Here's how the part is built. I have some questions about the finished solid (model axes, mm). A direction names the side the tool comes from. Give positions to 0.01 mm unless a question says otherwise; leave off trailing zeros. Loops run counter-clockwise (first coordinate to the right, second up) from the corner with the lowest first, then second, coordinate; pieces in that order, holes last.
Q1. I need wall thicknesses on probe 1 along X at (y, z) = (-45, -8); probe 2 along Y at (x, z) = (41, -0.5); probe 3 along Z at (x, y) = (-34, 45). Which ranges of each line are inside material? Lowest first, please.
Q2. Suppose I cut it at A-A (y = -44). List the corners of the cut face in (x, z) for me, and give its area (3 significant figures).
Q3. I'm going to push flat-ended pins straight in: P1, Ø7, axis at y = 15.5, z = -0.5, coming from the +X side; P2, Ø10, axis at x = -50, y = 1.5, coming from the +Z side; P3, Ø6.5, axis at y = -75.5, z = 1, coming from the -X side. Where does each tip first touch, or does it pass through?
Q4. Thinking about a two-plate mould opening in Y: for faces 1 (the face through (69.85, -76, 0)), 2 (the face through (57.15, 15, 0)), 3 (the face through (67.63, -74.75, -12.28)), 4 (the face through (1.2, 61.1, -5.6)), which applies, pulls with the +Y half, pulls with the -Y half, needs draft (parallel to the pull), parting line crosses it, or undercut?
Q5. For faces 5 (the face through (34.436, -78.468, -1.816)), 6 (the face through (58.402, 12.9, 2.146)), 7 (the face through (0.212, -74.751, -23.872)), 8 (the face through (-69.02, -36.06, -23.95)), 9 (the face through (-1, -63.5, -6)), which set-ups out of +Z, -Z, +X, -X, +Y, -Y let a thin tool reach every point of the face, with its end or its side?
```python
from build123d import *

# Parameters (mm, degrees)
F4_DEPTH       = 25.4
F1_R           = 6.35
F5_DEPTH       = 69.85
F3_R           = 6.604
F6_DEPTH       = 69.85
F7_R           = 5.07999
F2_R           = 2.9845
F8_DEPTH       = 69.85
F10_DEPTH      = 11.43
F12_DEPTH      = 25.4
F12_DEPTH_BACK = 25.4
F13_R          = 3.175
F14_DEPTH      = 59.69
F14_DEPTH_BACK = 59.69
F15_R          = 3.1877
F16_DEPTH      = 57.15
F16_DEPTH_BACK = 57.15


# Not quite as in the source:
# - a fillet or chamfer is up to 0.001 mm smaller than in the source, because OpenCascade refuses the exact size


with BuildPart() as f4:
    # F0 (on Top) → F4 (new body)
    with BuildSketch(Plane.XY):
        with BuildLine():
            Line((69.1548068551, -76.2), (69.1548068551, 0))
            ThreePointArc((69.1548068551, 0), (-0.6951931449, 69.85), (-70.5451931449, 0))
            Line((-70.5451931449, 0), (-70.5451931449, -76.2))
            Line((-70.5451931449, -76.2), (69.1548068551, -76.2))
        make_face()
    extrude(amount=-F4_DEPTH)

    # F1 (on Right) → F5 (join)
    with BuildSketch(Plane.YZ):
        with Locations((-76.4005258679, 0)):
            Circle(F1_R)
    extrude(amount=-F5_DEPTH)

    # F3 (on Right) → F6 (cut)
    with BuildSketch(Plane.YZ):
        with Locations((-76.365634799, 0)):
            Circle(F3_R)
    extrude(amount=F6_DEPTH, mode=Mode.SUBTRACT)

    # F7 (radius 5.08 in the source; OpenCascade refuses exactly that, so slightly less here)
    f7_edges = [f4.edges().sort_by_distance(p)[0] for p in [
        (-0.695193, -76.2, -25.4),
        (-70.545193, -38.1, -25.4),
        (-70.545193, -76.2, -12.7),
        (69.154807, -76.2, -16.000961),
    ]]
    fillet(f7_edges, radius=F7_R)

    # F2 (on Right) → F8 (join)
    with BuildSketch(Plane.YZ):
        with Locations((-76.0997384787, 0)):
            Circle(F2_R)
    extrude(amount=F8_DEPTH)

    # F9 (on Top) → F10 (cut)
    with BuildSketch(Plane.XY):
        with BuildLine():
            Line((60.994354069, -63.5), (60.994354069, 0))
            ThreePointArc((60.994354069, 0), (-0.118045931, 61.1124), (-61.230445931, 0))
            Line((-61.230445931, 0), (-61.230445931, -63.5))
            Line((-61.230445931, -63.5), (60.994354069, -63.5))
        make_face()
    extrude(amount=-F10_DEPTH, mode=Mode.SUBTRACT)

    # F11 (on Right) → F12 (cut, two sides)
    with BuildSketch(Plane.YZ) as f12_sk:
        Polygon((71.3768934982, -16.6989553797), (69.8592278852, 0), (69.8592278852, -4.7290348448), (65.7952278852, -4.7290348448), align=None)
    extrude(amount=-F12_DEPTH, mode=Mode.SUBTRACT)
    extrude(f12_sk.sketch, amount=F12_DEPTH_BACK, mode=Mode.SUBTRACT)

    # F13 (on Right) → F14 (join, two sides)
    with BuildSketch(Plane.YZ) as f14_sk:
        with Locations((15.24, 0)):
            Circle(F13_R)
    extrude(amount=F14_DEPTH)
    extrude(f14_sk.sketch, amount=-F14_DEPTH_BACK)

    # F15 (on Right) → F16 (cut, two sides)
    with BuildSketch(Plane.YZ) as f16_sk:
        with Locations((15.24, 0)):
            Circle(F15_R)
    extrude(amount=-F16_DEPTH, mode=Mode.SUBTRACT)
    extrude(f16_sk.sketch, amount=F16_DEPTH_BACK, mode=Mode.SUBTRACT)


solid = f4.part
```
Solutions:
1. probe 1: x = -70.55 to -61.23, 60.99 to 69.15
1. probe 2: y = -79.04 to -73.16, -69.78 to -63.5, 45.21 to 56.04
1. probe 3: z = -25.4 to -11.43
2. outline: (-70.55, -20.32) arc R5.08 ccw to (-65.47, -25.4) - (64.07, -25.4) arc R5.08 ccw to (69.15, -20.32) - (69.15, 0) - (60.99, 0) - (60.99, -11.43) - (-61.23, -11.43) - (-61.23, 0) - (-70.55, 0) - close
2. area: 2,140 mm2
3. P1: stops at x = 68.12
3. P2: stops at z = -11.43
3. P3: stops at x = -70.38
4. face 1: needs draft
4. face 2: undercut
4. face 3: pulls with the -Y half
4. face 4: undercut
5. face 5: +X
5. face 6: none
5. face 7: -Z, +X, -X, -Y
5. face 8: -Z, -X, +Y, -Y
5. face 9: +Z
